Geometry: final body of the model. Coordinates: model frame, mm. A direction names the side the tool comes from. Coordinates: 2 decimals unless noted, no trailing zeros. Order: outer loops, then holes, each group sorted by start corner. A loop starts at its lowest first (then second) coordinate and runs counter-clockwise, first axis right, second up. Notation, with made-up numbers: M 76.25,-36 L 85.25,-36 A13 ccw 85.25,-19 Z; hole C 16.25,-3.75 d1. An arc over 180 degrees is marked long. Write item = value, one per line.
from build123d import *

# Parameters (mm, degrees)
CENTER_BODY_DEPTH               = 10
SKETCH1_3_R                     = 1.6
SKETCH1_3_R_2                   = 1.6000000000000003
CONNECTOR_BODY_DEPTH            = 5
MECH_LOCK_LEFT_DEPTH            = 5
DULLING_FILLET_GENERAL_R        = 0.5
ELEPHANTSFOOT_COMPENSATION_SIZE = 0.5
DULLING_FILLET_LEFT_R           = 0.5


with BuildPart() as part:
    # complete_sketch → center_body (new body)
    with BuildSketch(Plane(origin=(0, 0, 0), x_dir=(1, 0, 0), z_dir=(0, 1, 0))):
        Polygon((-5, 47), (-5, 5.958767962971026), (5, 4.195498155886416), (5, 47), align=None)
    extrude(amount=CENTER_BODY_DEPTH)

    # Sketch1_3 → connector_body (add)
    # profile 1 of 2: a face of its own
    with BuildSketch(Plane(origin=(0, 0, 0), x_dir=(1, 0, 0), z_dir=(0, 1, 0))):
        with BuildLine():
            Line((-5, 5.958767962971026), (-5, 0))
            ThreePointArc((-5, 0), (-3.1e-16, -5), (5, -6.1e-16))
            Line((5, 0), (5, 4.195498155886416))
            Line((5, 4.195498155886416), (-5, 5.958767962971026))
        make_face()
        with Locations(Location((0, 0, 0), (0, 0, 270))):
            Circle(SKETCH1_3_R, mode=Mode.SUBTRACT)
    # profile 2 of 2: a face of its own
    with BuildSketch(Plane(origin=(0, 0, 0), x_dir=(1, 0, 0), z_dir=(0, 1, 0))):
        with BuildLine():
            Line((-5, 52.70871215252208), (-5, 47))
            Line((-5, 47), (5, 47))
            Line((5, 47), (5, 52.70871215252208))
            Line((5, 52.70871215252208), (5, 55))
            ThreePointArc((5, 55), (-1.4e-16, 60), (-5, 55))
            Line((-5, 55), (-5, 52.70871215252208))
        make_face()
        with Locations(Location((0, 55, 0), (0, 0, 270))):
            Circle(SKETCH1_3_R_2, mode=Mode.SUBTRACT)
    extrude(amount=CONNECTOR_BODY_DEPTH)

    # Sketch1 → mech_lock_left (add)
    with BuildSketch(Plane(origin=(0, 5, 0), x_dir=(1, 0, 0), z_dir=(0, 1, 0))):
        with BuildLine():
            Line((-5, 47), (5, 47))
            Line((5, 47), (5, 55))
            ThreePointArc((5, 55), (3.535533905932735, 51.46446609406726), (0, 49.99999999999999))
            ThreePointArc((0, 49.99999999999999), (-2.637161951805669, 49.34290487951417), (-4.999999999999999, 48))
            Line((-4.999999999999999, 48), (-5, 47))
        make_face()
    extrude(amount=MECH_LOCK_LEFT_DEPTH)

    # dulling_fillet_general
    dulling_fillet_general_edges = [part.edges().sort_by_distance(p)[0] for p in [
        (5, 7.5, -4.195498155886416),
        (-5, 7.5, -5.958767962971026),
    ]]
    fillet(dulling_fillet_general_edges, radius=DULLING_FILLET_GENERAL_R)

    # elephantsfoot_compensation
    elephantsfoot_compensation_edges = [part.edges().sort_by_distance(p)[0] for p in [
        (1.4e-16, 0, 5),
        (4.9e-16, 0, -1.6),
        (-1.4e-16, 0, -60),
        (4.9e-16, 0, -56.6),
        (5, 0, -27.5),
        (-5, 0, -27.5),
    ]]
    chamfer(elephantsfoot_compensation_edges, length=ELEPHANTSFOOT_COMPENSATION_SIZE)

    # dulling_fillet_left
    dulling_fillet_left_edges = [part.edges().sort_by_distance(p)[0] for p in [
        (5, 7.5, -55),
    ]]
    fillet(dulling_fillet_left_edges, radius=DULLING_FILLET_LEFT_R)


solid = part.part
1) Section C-C, the plane y = 4. Return loops of the section in (x, z).
Numbers:
outline = M -5,-55 A5 ccw 5,-55 L 5,0 A5 ccw -5,0 Z; hole C 0,-55 d3.2; hole C 0,0 d3.2
2) Mould query, pull axis X, two halves, no side actions, for faces 4 (the face through (0.481, 2.718, -53.474)), 5 (the face through (0, 10, -29)), 6 (the face through (5, 5, -27)). Classes: pulls with the +X half, pulls with the -X half, needs draft (parallel to the pull), parting line crosses it, or undercut.
Numbers:
face_4 = undercut
face_5 = needs draft
face_6 = pulls with the +X half
3) Section B-B, the plane z = -3. Return loops of the section in (x, y).
Numbers:
outline = M -5,0.5 L -4.5,0 L 4.5,0 L 5,0.5 L 5,5 L -5,5 Z
4) Section A-A, the plane y = 7.25. Return loops of the section in (x, z), and give its area (3 significant figures).
Numbers:
outline = M -5,-48 A10 ccw 0,-50 A5 cw 4.09,-52.13 A0.5 ccw 5,-51.84 L 5,-4.79 A0.5 ccw 4.41,-4.3 L -4.59,-5.89 A0.5 ccw -5,-6.38 Z
area = 450 mm²
5) Set-up query: faces 1 (the face through (-0.15, 7.465, -5.104)), 2 (the face through (0, 3, -60)), 3 (the face through (2.335, 7.465, -50.579)). Return all of +Z, -Z, +X, -X, +Y, -Y with unobstructed straight access to the full face (end or side cutting, diameter ignored); none if empty.
Numbers:
face_1 = +Z, -X, +Y
face_2 = -Z, +Y, -Y
face_3 = -Z, -X, +Y
6) Pin query (flat end, axial travel): pin 1 (3 mm diameter, centred on x = 0.5, z = -2.5, fed in from +Y); pin 2 (1.5 mm diameter, centred on x = -1.5, y = 8.5, fed in from -Z). Return the tip coordinate at first contact, or that it passes through.
Numbers:
pin_1 = 5
pin_2 = -49.89
7) Section D-D, the plane z = -49. Return loops of the section in (x, y).
Numbers:
outline = M -5,0.5 L -4.5,0 L 4.5,0 L 5,0.5 L 5,10 L -3.4,10 L -3.4,5 L -5,5 Z
8) Line query: L1, parallel to Z at x = 0.25, y = 1; L2, parallel to Y at x = 0.25, z = -50.5; L3, parallel to Z at x = 1.5, y = 6. Output: solid intervals per line, ascending.
Numbers:
L1 = -59.99 to -56.58, -53.42 to -1.58, 1.58 to 4.99
L2 = 0 to 5
L3 = -50.23 to -4.81
